Part model, mm, in its own coordinate system. Face numbers are marked on the shaded views. A direction names the side the tool comes from. Round coordinates to 2 decimals unless told otherwise and drop trailing zeros. Write each loop counter-clockwise with the first axis right and the second up, starting at its lowest first coordinate (ties: lowest second). Pieces come first, ordered by that corner, then holes. Notation, with made-up numbers: M -40,-3 L 6,-3 A21 cw 6,4 Z; hole C -38,-27 d10. An arc over 180 degrees is marked long. Use one line per item in the form item = value. Start each with the question number.
Item 1: Cut at D-D, the plane y = 65. Give the cut face in (x, z).
Item 2: Cut at A-A, the plane z = 0. Give the cut face in (x, y).
Item 3: Cut at C-C, the plane y = -58. Give the cut face in (x, z), then the cut area to 3 significant figures.
Item 4: Which spindle directions (+Z, -Z, +X, -X, +Y, -Y) get a long thin tool onto all of the face, cutting with end or side? Do the marked faces 1 and 2. Say none if no direction does.
Item 5: Mould opens along Z. For the marked faces 3, 4, 5 and 6 say: +Z half, -Z half, draft (parallel to the pull), parting line (faces both ways), or undercut.
Item 6: Probe L1, parallel to Z at x = 23, y = -50; L2, parallel to Y at x = 54.5, z = 8; L3, parallel to Z at x = 3, y = 5. List the from-to ranges inside material, lowest first.
Item 7: Cut at B-B, the plane x = 33. Give the cut face in (y, z), then the cut area to 3 significant figures.
Item 8: Flat gauge pins, fed straight in: pin 1 Ø6 at (y, z) = (-20.5, 7.5) entering from +X; pin 2 Ø12 at (x, z) = (51, -23.5) entering from -Y; pin 3 Ø8 at (y, z) = (-4, -15) entering from -X. Where does each tip first touch, or does it go through?
from build123d import *

# Parameters (mm, degrees)
F0_W     = 100
F0_H     = 10
F1_DEPTH = 60
F2_START = 5
F0_H_2   = 40
F2_DEPTH = 50
F3_R     = 10
F4_DEPTH = 55.001


with BuildPart() as f1:
    # F0 (on Right) → F1 (new body)
    with BuildSketch(Plane.YZ):
        with Locations((0, 25)):
            Rectangle(F0_W, F0_H)
        with BuildLine():
            Line((-50, 20), (-50, 30))
            ThreePointArc((-50, 30), (-80, 0), (-50, -30))
            Line((-50, -30), (-50, -20))
            ThreePointArc((-50, -20), (-70, 0), (-50, 20))
        make_face()
        with BuildLine():
            ThreePointArc((50, -30), (80, 0), (50, 30))
            Line((50, 30), (50, 20))
            ThreePointArc((50, 20), (70, 0), (50, -20))
            Line((50, -20), (50, -30))
        make_face()
        with Locations((0, -25)):
            Rectangle(F0_W, F0_H)
    extrude(amount=F1_DEPTH)

    # F0 (on Right) → F2 (join)
    with BuildSketch(Plane.YZ.offset(F2_START)):
        Rectangle(F0_W, F0_H_2)
        with BuildLine():
            ThreePointArc((50, -20), (70, 0), (50, 20))
            Line((50, 20), (50, -20))
        make_face()
        with BuildLine():
            Line((-50, -20), (-50, 20))
            ThreePointArc((-50, 20), (-70, 0), (-50, -20))
        make_face()
    extrude(amount=F2_DEPTH)

    # F3 (on face) → F4 (cut, through all)
    with BuildSketch(Plane.YZ.offset(55)):
        with Locations((-50, 0)):
            Circle(F3_R)
        with Locations((50, 0)):
            Circle(F3_R)
    extrude(amount=-F4_DEPTH, mode=Mode.SUBTRACT)


solid = f1.part
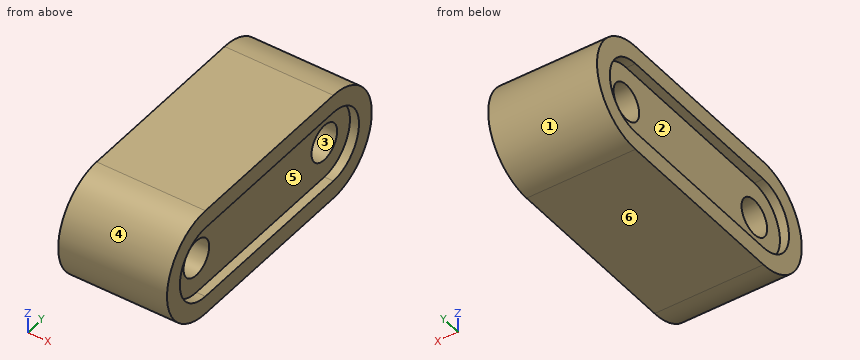
Model answer:
q1.outline = M 0,-25.98 L 60,-25.98 L 60,-13.23 L 55,-13.23 L 55,13.23 L 60,13.23 L 60,25.98 L 0,25.98 L 0,13.23 L 5,13.23 L 5,-13.23 L 0,-13.23 Z
q2.outline = M 0,-80 L 60,-80 L 60,-70 L 55,-70 L 55,-60 L 5,-60 L 5,-70 L 0,-70 Z; M 0,70 L 5,70 L 5,60 L 55,60 L 55,70 L 60,70 L 60,80 L 0,80 Z; M 5,-40 L 55,-40 L 55,40 L 5,40 Z
q3.outline = M 0,-28.91 L 60,-28.91 L 60,-18.33 L 55,-18.33 L 55,-6 L 5,-6 L 5,-18.33 L 0,-18.33 Z; M 0,18.33 L 5,18.33 L 5,6 L 55,6 L 55,18.33 L 60,18.33 L 60,28.91 L 0,28.91 Z
q3.area = 2,500 mm²
q4.face_1 = +X, -X, +Y
q4.face_2 = -X
q5.face_3 = undercut
q5.face_4 = parting line
q5.face_5 = undercut
q5.face_6 = -Z half
q6.L1 = -30 to -10, 10 to 30
q6.L2 = -78.91 to -56, -44 to 44, 56 to 78.91
q6.L3 = -30 to -20, 20 to 30
q7.outline = M -50,-30 L 50,-30 A30 ccw 50,30 L -50,30 A30 ccw Z; hole C -50,0 d20; hole C 50,0 d20
q7.area = 8,200 mm²
q8.pin_1 = 55
q8.pin_2 = -74.37
q8.pin_3 = 5
